For this review, take the finished solid that the model builds, in its own axes (mm). Face numbers are marked on the shaded views. A direction names the side the tool comes from. Give positions to 0.01 mm unless a question says otherwise; leave off trailing zeros. Loops run counter-clockwise (first coordinate to the right, second up) from the corner with the lowest first, then second, coordinate; pieces in that order, holes last. Notation, with made-up numbers: (5.5, 69.5) -> (55.5, 69.5) arc R12 cw to (55.5, 88.5) -> close; hole circle Ø11 at (-22.5, -15.75). An arc over 180 degrees is marked (long way). Write each question's results on one line, items separated by ' | '. Start each with the question number.
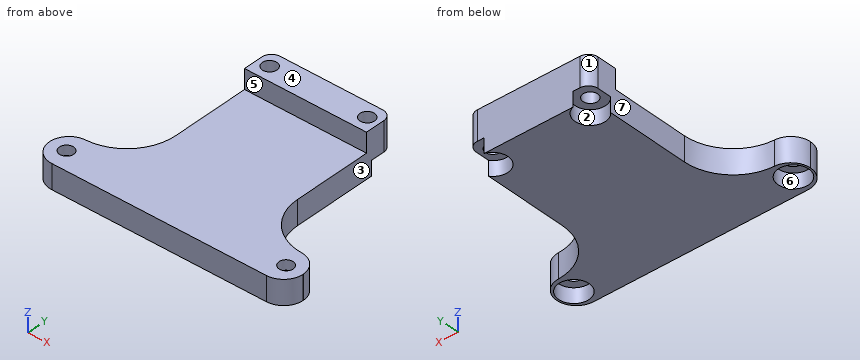
```python
from build123d import *

# Parameters (mm, degrees)
SKETCH_1_W          = 52
SKETCH_1_H          = 8
SKETCH_1_R          = 1.45
EXTRUDE_1_DEPTH     = 5
SKETCH_2_W          = 25
SKETCH_2_H          = 32
SKETCH_2_R          = 1.5
EXTRUDE_2_DEPTH     = 5
SKETCH_3_W          = 25
SKETCH_3_H          = 6
SKETCH_3_R          = 1.5
EXTRUDE_3_DEPTH     = 4
FILLET_1_R          = 10
FILLET_2_R          = 4
FILLET_3_R          = 2
SKETCH_4_R          = 3.125
CUT_EXTRUDE_3_DEPTH = 3


with BuildPart() as part:
    # Эскиз1 → Бобышка-Вытянуть1 (new body)
    with BuildSketch(Plane.XY):
        Rectangle(SKETCH_1_W, SKETCH_1_H)
        with Locations((-22.5, 0)):
            Circle(SKETCH_1_R, mode=Mode.SUBTRACT)
        with Locations((22.5, 0)):
            Circle(SKETCH_1_R, mode=Mode.SUBTRACT)
    extrude(amount=EXTRUDE_1_DEPTH)

    # Эскиз2 → Бобышка-Вытянуть2 (add)
    with BuildSketch(Plane(origin=(0, 0, 0), x_dir=(-1, 0, 0), z_dir=(0, 0, -1))):
        with Locations((0, 20)):
            Rectangle(SKETCH_2_W, SKETCH_2_H)
        with Locations((-10, 33)):
            Circle(SKETCH_2_R, mode=Mode.SUBTRACT)
        with Locations((10, 33)):
            Circle(SKETCH_2_R, mode=Mode.SUBTRACT)
    extrude(amount=-EXTRUDE_2_DEPTH)

    # Эскиз3 → Бобышка-Вытянуть3 (add)
    with BuildSketch(Plane(origin=(0, 0, 5), x_dir=(-1, 0, 0), z_dir=(0, 0, -1))):
        with Locations((0, 33)):
            Rectangle(SKETCH_3_W, SKETCH_3_H)
        with Locations((10, 33)):
            Circle(SKETCH_3_R, mode=Mode.SUBTRACT)
        with Locations((-10, 33)):
            Circle(SKETCH_3_R, mode=Mode.SUBTRACT)
    extrude(amount=-EXTRUDE_3_DEPTH)

    # Скругление1
    fillet_1_edges = [part.edges().sort_by_distance(p)[0] for p in [
        (12.5, 4, 2.5),
        (-12.5, 4, 2.5),
    ]]
    fillet(fillet_1_edges, radius=FILLET_1_R)

    # Скругление2
    fillet_2_edges = [part.edges().sort_by_distance(p)[0] for p in [
        (-26, -4, 2.5),
        (-26, 4, 2.5),
        (26, -4, 2.5),
        (26, 4, 2.5),
    ]]
    fillet(fillet_2_edges, radius=FILLET_2_R)

    # Скругление3
    fillet_3_edges = [part.edges().sort_by_distance(p)[0] for p in [
        (12.5, 36, 4.5),
        (-12.5, 36, 4.5),
    ]]
    fillet(fillet_3_edges, radius=FILLET_3_R)

    # Эскиз4 → Вырез-Вытянуть3 (cut)
    with BuildSketch(Plane(origin=(0, 0, 0), x_dir=(-1, 0, 0), z_dir=(0, 0, -1))):
        with Locations((-10, 33)):
            Circle(SKETCH_4_R)
        with Locations((10, 33)):
            Circle(SKETCH_4_R)
        with Locations((-22.5, 0)):
            Circle(SKETCH_4_R)
        with Locations((22.5, 0)):
            Circle(SKETCH_4_R)
    extrude(amount=-CUT_EXTRUDE_3_DEPTH, mode=Mode.SUBTRACT)


solid = part.part
```
1. For pin 1 Ø6 at (x, y) = (14.5, 6.5) entering from +Z; pin 2 Ø3 at (x, y) = (22.5, -0.5) entering from -Z; pin 3 Ø2.5 at (y, z) = (22.5, 5.5) entering from +X, all flat-tipped, find the tip position at first contact; note any pin that passes through.
2. Machinability: for the marked faces 4, 5, 6 and 7, which of the approach directions +Z, -Z, +X, -X, +Y, -Y give a long, thin tool a straight path to every point of the face, cutting with its end or side? Answer none if there is none.
3. We need section C-C (x = -3.5). Write out the cut boundary in (y, z), plus the area to 3 significant figures.
4. Wall thickness on L1, parallel to X at y = 0, z = 3.6; L2, parallel to X at y = 2, z = 1.75; L3, parallel to Z at x = -7.5, y = 27.5: over which ranges is each line inside the solid? List them lowest first.
5. Draft analysis for pull direction Y (two halves, no side actions). For the marked faces 1, 2 and 3, state which applies: released by +Y, released by -Y, zero draft, split by the parting line, or undercut.
6. We need section D-D (y = 21.5). Write out the cut boundary in (x, z).
7. We need section B-B (z = 7.5). Write out the cut boundary in (x, y), plus the area to 3 significant figures.
8. We need section A-A (y = 33). Write out the cut boundary in (x, z) (3 decimals).
Response:
1) pin 1: stops at z = 5 | pin 2: stops at z = 3 | pin 3: stops at x = 12.5
2) face 4: +Z, +X, -X, +Y, -Y | face 5: +Z, +X, -X, -Y | face 6: -Z | face 7: +Z, -Z, -X, +Y
3) outline: (-4, 0) -> (36, 0) -> (36, 9) -> (30, 9) -> (30, 5) -> (-4, 5) -> close | area: 224 mm2
4) L1: x = -26 to -23.95, -21.05 to 21.05, 23.95 to 26 | L2: x = -25.47 to -24.9, -20.1 to 20.1, 24.9 to 25.47 | L3: z = 0 to 5
5) face 1: released by +Y | face 2: undercut | face 3: zero draft
6) outline: (-12.5, 0) -> (12.5, 0) -> (12.5, 5) -> (-12.5, 5) -> close
7) outline: (-12.5, 30) -> (12.5, 30) -> (12.5, 34) arc R2 ccw to (10.5, 36) -> (-10.5, 36) arc R2 ccw to (-12.5, 34) -> close; hole circle Ø3 at (-10, 33); hole circle Ø3 at (10, 33) | area: 134 mm2
8) outline: (-12.5, 3) -> (-11.5, 3) -> (-11.5, 9) -> (-12.5, 9) -> close; (-8.5, 3) -> (-6.875, 3) -> (-6.875, 0) -> (6.875, 0) -> (6.875, 3) -> (8.5, 3) -> (8.5, 9) -> (-8.5, 9) -> close; (11.5, 3) -> (12.5, 3) -> (12.5, 9) -> (11.5, 9) -> close
